from build123d import *

# Parameters (mm, degrees)
SKETCH_1_W          = 40.5
SKETCH_1_H          = 20
EXTRUDE_1_DEPTH     = 28
SKETCH_2_W          = 7.75
SKETCH_2_H          = 20
SKETCH_2_W_2        = 40.5
EXTRUDE_2_DEPTH     = 2.5
SKETCH_3_W          = 40.5
SKETCH_3_H          = 20
EXTRUDE_3_DEPTH     = 12
SKETCH_4_R          = 3
EXTRUDE_4_DEPTH     = 4
SKETCH_5_R          = 1.65
CUT_EXTRUDE_1_DEPTH = 61.483985484


with BuildPart() as part:
    # 草图1 → 凸台-拉伸1 (new body)
    with BuildSketch(Plane.XY):
        with Locations((20.25, -10)):
            Rectangle(SKETCH_1_W, SKETCH_1_H)
    extrude(amount=EXTRUDE_1_DEPTH)

    # 草图2 → 凸台-拉伸2 (add)
    with BuildSketch(Plane.XY.offset(28)):
        with Locations((-3.875, -10)):
            Rectangle(SKETCH_2_W, SKETCH_2_H)
        with Locations((20.25, -10)):
            Rectangle(SKETCH_2_W_2, SKETCH_2_H)
        with Locations((44.375, -10)):
            Rectangle(SKETCH_2_W, SKETCH_2_H)
    extrude(amount=EXTRUDE_2_DEPTH)

    # 草图3 → 凸台-拉伸3 (add)
    with BuildSketch(Plane.XY.offset(30.5)):
        with Locations((20.25, -10)):
            Rectangle(SKETCH_3_W, SKETCH_3_H)
    extrude(amount=EXTRUDE_3_DEPTH)

    # 草图4 → 凸台-拉伸4 (add)
    with BuildSketch(Plane.XY.offset(42.5)):
        with Locations((30, -10)):
            Circle(SKETCH_4_R)
    extrude(amount=EXTRUDE_4_DEPTH)

    # 草图5 → 切除-拉伸1 (cut, through all)
    with BuildSketch(Plane.XY.offset(30.5)):
        with Locations((-3.75, -5)):
            Circle(SKETCH_5_R)
        with Locations((-3.75, -15)):
            Circle(SKETCH_5_R)
        with Locations((44.25, -5)):
            Circle(SKETCH_5_R)
        with Locations((44.25, -15)):
            Circle(SKETCH_5_R)
    extrude(amount=-CUT_EXTRUDE_1_DEPTH, mode=Mode.SUBTRACT)


solid = part.part
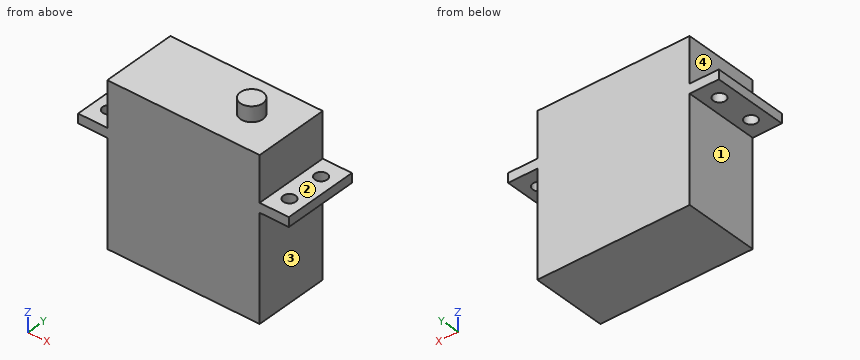
For this review, take the finished solid that the model builds, in its own axes (mm). Face numbers are marked on the shaded views. A direction names the side the tool comes from. Round coordinates to 2 decimals unless told otherwise and drop trailing zeros. Loops run counter-clockwise (first coordinate to the right, second up) from the corner with the lowest first, then second, coordinate; pieces in that order, holes last. Notation, with made-up numbers: (67.5, -33.75) - (81.5, -33.75) arc R14 cw to (81.5, -27.75) - close; hole circle Ø1 at (-23, 54.25). An arc over 180 degrees is marked (long way). Use one line per item in the form item = value.
Item 1: Clearance check with flat-ended pins moving along their axes: P1, Ø2.5, axis at x = -3.75, y = -15, coming from the -Z side; P2, Ø4, axis at x = -5, y = -7, coming from the -Z side; P3, Ø1, axis at x = 4.5, z = 12.5, coming from the +Y side; P4, Ø6, axis at x = 20.5, y = -9.5, coming from the +Z side. State where each tip first meets the part, or that it passes through.
Answers:
P1 = through
P2 = 28
P3 = 0
P4 = 42.5
Item 2: Tool access review of the marked faces 1, 2, 3 and 4: name each direction out of +Z, -Z, +X, -X, +Y, -Y from which nothing blocks a thin tool from reaching the whole face with its end or side.
Answers:
face_1 = -Z, -X, +Y, -Y
face_2 = +Z, +X, +Y, -Y
face_3 = -Z, +X, +Y, -Y
face_4 = +Z, -X, +Y, -Y
Item 3: Consider section C-C on x = 30. Write out the cut boundary in (y, z), then the cut area to 3 significant figures.
Answers:
outline = (-20, 0) - (0, 0) - (0, 42.5) - (-7, 42.5) - (-7, 46.5) - (-13, 46.5) - (-13, 42.5) - (-20, 42.5) - close
area = 874 mm^2
Item 4: Consider section B-B on x = 44.25. Write out the cut boundary in (y, z).
Answers:
outline = (-20, 28) - (-16.65, 28) - (-16.65, 30.5) - (-20, 30.5) - close; (-13.35, 28) - (-6.65, 28) - (-6.65, 30.5) - (-13.35, 30.5) - close; (-3.35, 28) - (0, 28) - (0, 30.5) - (-3.35, 30.5) - close
Item 5: For line 1 (Y direction, x = 44.25, z = 28.55); line 2 (Z direction, x = 7, y = -8); line 3 (X direction, y = -10.75, z = 6), list the stretches that pass through material, from the lowest coordinate up.
Answers:
line_1 = -20 to -16.65, -13.35 to -6.65, -3.35 to 0
line_2 = 0 to 42.5
line_3 = 0 to 40.5
Item 6: Consider section A-A on y = -5. Write out the cut boundary in (x, z).
Answers:
outline = (-7.75, 28) - (-5.4, 28) - (-5.4, 30.5) - (-7.75, 30.5) - close; (-2.1, 28) - (0, 28) - (0, 0) - (40.5, 0) - (40.5, 28) - (42.6, 28) - (42.6, 30.5) - (40.5, 30.5) - (40.5, 42.5) - (0, 42.5) - (0, 30.5) - (-2.1, 30.5) - close; (45.9, 28) - (48.25, 28) - (48.25, 30.5) - (45.9, 30.5) - close
Item 7: Consider section D-D on y = -10. Write out the cut boundary in (x, z).
Answers:
outline = (-7.75, 28) - (0, 28) - (0, 0) - (40.5, 0) - (40.5, 28) - (48.25, 28) - (48.25, 30.5) - (40.5, 30.5) - (40.5, 42.5) - (33, 42.5) - (33, 46.5) - (27, 46.5) - (27, 42.5) - (0, 42.5) - (0, 30.5) - (-7.75, 30.5) - close
